Verification items for the finished model (mm, model axes). Coordinates: 2 decimals unless noted, no trailing zeros. Order: outer loops, then holes, each group sorted by start corner. A loop starts at its lowest first (then second) coordinate and runs counter-clockwise, first axis right, second up. Notation, with made-up numbers: M 5.5,66 L 17.5,66 A24 ccw 17.5,87 Z; hole C 75.25,9.5 d5. An arc over 180 degrees is marked long. Write item = value, one per line.
Autodesk Inventor part; units mm, degrees
ref_plane "YZ Plane" through (0, 0, 0) normal (1, 0, 0) x (0, 1, 0)
ref_plane "XZ Plane" through (0, 0, 0) normal (0, 1, 0) x (-1, 0, 0)
ref_plane "XY Plane" through (0, 0, 0) normal (0, 0, 1) x (1, 0, 0)
sketch "Sketch1" plane through (0, 0, 0) normal (0, 0, 1) x (1, 0, 0)
  line L0 (-21.1568, 46.0602) -> (29.6432, 46.0602)
  line L1 (29.6432, 46.0602) -> (29.6432, -4.7398)
  line L2 (29.6432, -4.7398) -> (26.4682, -4.7398)
  line L3 (-21.1568, 42.8852) -> (-21.1568, 46.0602)
  line L4 (-21.1568, 42.8852) -> (26.4682, 42.8852)
  line L5 (26.4682, 42.8852) -> (26.4682, -4.7398)
  dimension "d0" = 50.8
  dimension "d1" = 50.8
  dimension "d2" = 3.175
  dimension "d3" = 3.175
extrude "Extrusion1" add sketch "Sketch1" along normal blind 1812.925
sketch "Sketch2" plane through (26.4682, -4.7398, 0) normal (-1, 0, 0) x (0, 0, 1)
  circle A0 centre (37.3062, 12.7) radius 10.3188
  circle A1 centre (93.6625, 17.4625) radius 7.1437
  line L0 (0, 50.8) -> (1812.925, 50.8)
  circle A2 centre (550.8625, 17.4625) radius 7.1437
  circle A3 centre (957.2625, 17.4625) radius 7.1437
  circle A4 centre (1363.6625, 17.4625) radius 7.1437
  circle A5 centre (1719.2625, 17.4625) radius 7.1437
  circle A6 centre (1775.6187, 12.7) radius 10.3188
  line L1 (1812.925, 0) -> (1812.925, 47.625)
  dimension "d8" = 20.6375
  dimension "d9" = 14.2875
  dimension "d12" = 38.1
  dimension "d13" = 33.3375
  dimension "d14" = 14.2875
  dimension "d15" = 14.2875
  dimension "d16" = 14.2875
  dimension "d17" = 14.2875
  dimension "d25" = 20.6375
  dimension "d26" = 38.1
  dimension "d27" = 37.3062
  dimension "d28" = 93.6625
  dimension "d29" = 449.2625
  dimension "d30" = 855.6625
  dimension "d31" = 1262.0625
  dimension "d32" = 1719.2625
  dimension "d33" = 1775.6188
extrude "Extrusion2" cut sketch "Sketch2" against normal blind 1812.925
equation "\"d14\" = d9"
equation "\"d15\" = d9"
equation "\"d16\" = d9"
equation "\"d17\" = d9"
equation "\"d25\" = d8"
equation "\"d26\" = d12"
properties part number "FE-00007-01"
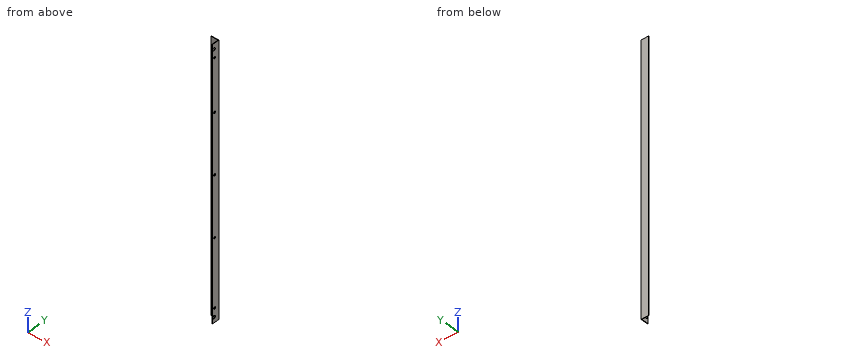
Item 1: Scan lines: L1, parallel to X at y = -2, z = 1141.5; L2, parallel to Y at x = 22.5, z = 426.5. Record each from-to range of solid material in increasing order. Write a range as from..to.
Report:
L1 = 26.47..29.64
L2 = 42.89..46.06
Item 2: Sectioned sample at C-C, the plane y = 31. Enter the section's corners in (x, z) (3 decimals).
Report:
outline = M 26.468,0 L 29.643,0 L 29.643,1812.925 L 26.468,1812.925 Z
Item 3: Sectioned sample at A-A, the plane z = 1206. Enter the section's corners in (x, y), then the cut area to 4 significant figures.
Report:
outline = M -21.16,42.89 L 26.47,42.89 L 26.47,-4.74 L 29.64,-4.74 L 29.64,46.06 L -21.16,46.06 Z
area = 312.5 mm^2
Item 4: Gauge pin test, flat end, axial feed: pin 1 (5 mm diameter, centred on y = 36.5, z = 569.5, fed in from -X). Record the tip position at first contact, or that the pin passes through.
Report:
pin_1 = 26.47
Item 5: Sectioned sample at B-B, the plane x = -6. Enter the section's corners in (y, z) (3 decimals), then the cut area to 3 significant figures.
Report:
outline = M 42.885,0 L 46.06,0 L 46.06,1812.925 L 42.885,1812.925 Z
area = 5,760 mm^2
